Autodesk Inventor part; units mm, degrees
ref_plane "YZ Plane" through (0, 0, 0) normal (1, 0, 0) x (0, 1, 0)
ref_plane "XZ Plane" through (0, 0, 0) normal (0, 1, 0) x (-1, 0, 0)
ref_plane "XY Plane" through (0, 0, 0) normal (0, 0, 1) x (1, 0, 0)
ref_plane "Work Plane2" through (35.545, -31.609, 1.6) normal (0, 0, 1) x (1, 0, 0)
ref_plane "Work Plane1" through (35.545, -31.609, 1.6) normal (0, 0, 1) x (1, 0, 0)
sketch "Sketch1" plane through (35.545, -31.609, 1.6) normal (0, 0, 1) x (1, 0, 0)
  line L0 (0, 0) -> (336, 0)
  line L1 (-2, -129) -> (-2, -2)
  line L2 (-1.6825, -0.9187) -> (-1.5115, -0.6903)
  arc A0 (0, 0) -> (-2, -2) centre (0, -2) ccw
  line L3 (338, -2) -> (338, -129)
  line L4 (337.5115, -0.6903) -> (337.6825, -0.9187)
  arc A1 (338, -2) -> (336, 0) centre (336, -2) ccw
  line L5 (336, -131) -> (0, -131)
  line L6 (337.6825, -130.0813) -> (337.5115, -130.3097)
  arc A2 (336, -131) -> (338, -129) centre (336, -129) ccw
  arc A3 (-2, -129) -> (0, -131) centre (0, -129) ccw
  circle A4 centre (1.98, -128.63) radius 1.1
  circle A5 centre (1.98, -128.63) radius 1.1
  circle A6 centre (68.313, -128.63) radius 1.1
  circle A7 centre (134.646, -128.63) radius 1.1
  circle A8 centre (134.646, -128.63) radius 1.1
  circle A9 centre (68.313, -128.63) radius 1.1
  circle A10 centre (200.979, -128.63) radius 1.1
  circle A11 centre (267.312, -128.63) radius 1.1
  circle A12 centre (333.645, -128.63) radius 1.1
  circle A13 centre (333.645, -128.63) radius 1.1
  circle A14 centre (267.312, -128.63) radius 1.1
  circle A15 centre (200.979, -128.63) radius 1.1
  circle A16 centre (333.638, -2.355) radius 1.1
  circle A17 centre (1.973, -2.355) radius 1.1
  circle A18 centre (68.306, -2.355) radius 1.1
  circle A19 centre (134.639, -2.355) radius 1.1
  circle A20 centre (200.972, -2.355) radius 1.1
  circle A21 centre (267.305, -2.355) radius 1.1
  circle A22 centre (333.645, -2.355) radius 1.093
  circle A23 centre (267.305, -2.355) radius 1.1
  circle A24 centre (200.972, -2.355) radius 1.1
  circle A25 centre (134.639, -2.355) radius 1.1
  circle A26 centre (68.306, -2.355) radius 1.1
  circle A27 centre (1.973, -2.355) radius 1.1
  line L7 (3, -4.2357) -> (125.2758, -4.2357) construction
  line L8 (4, -5) -> (332, -5)
  line L9 (333, -6) -> (333, -125)
  line L10 (332, -126) -> (4, -126)
  line L11 (3, -125) -> (3, -6)
  arc A28 (4, -5) -> (3, -6) centre (4, -6) ccw
  arc A29 (333, -6) -> (332, -5) centre (332, -6) ccw
  arc A30 (332, -126) -> (333, -125) centre (332, -125) ccw
  arc A31 (3, -125) -> (4, -126) centre (4, -125) ccw
  line L12 (162.5077, 0) -> (162.5077, -5)
  line L13 (173.4174, -5) -> (173.4174, 0)
  circle A32 centre (320.737, -95.692) radius 0.175
  line L14 (333, -88.192) -> (338, -88.192)
  line L15 (333, -102.192) -> (338, -102.192)
  line L16 (257.6125, -126) -> (315.0362, -126)
  line L17 (315.0362, -126) -> (315.0362, -126.7604)
  line L18 (315.0362, -126.7604) -> (257.6125, -126.7604)
  line L19 (257.6125, -126.7604) -> (257.6125, -126)
  point P0 (-35.545, 31.609)
  point P1 (-1.5115, -130.3097)
  point P2 (335.5, -88.192)
  point P3 (0, -131)
  point P4 (337.6825, -130.0813)
  point P5 (-1.6825, -0.9187)
  point P6 (337.6825, -0.9187)
  dimension "d2" = 5
  dimension "d3" = 5
  dimension "d4" = 5
  dimension "d5" = 5
  dimension "d6" = 1
  dimension "d7" = 1
  dimension "d8" = 1
  dimension "d9" = 1
extrude "Extrusion3" add sketch "Sketch1" along normal blind 4.5 contours L0 A1 L4 L3 L14 L9 A29 L8 L13
properties part number "open_liner_S"
Here's how the part is built. I have some questions about the finished solid (model axes, mm). A direction names the side the tool comes from. Round coordinates to 2 decimals unless told otherwise and drop trailing zeros. Order: outer loops, then holes, each group sorted by start corner. A loop starts at its lowest first (then second) coordinate and runs counter-clockwise, first axis right, second up. Notation, with made-up numbers: M -4.5,17.25 L 3.5,17.25 A17 ccw 3.5,36.25 Z; hole C 77,-23.5 d6. An arc over 180 degrees is marked long. One line per question, with ' | ' between items.
1) I want a section at A-A, the plane z = 3.8. State how many separate pieces and enclosed holes the cut face has, then the cut area to 3 significant figures.
Working result:
separate pieces: 1 | enclosed holes: 3 | area: 1,230 mm²
2) I need wall thicknesses on line 1 along Y through (x, z) = (279, 4.9); line 2 along X through (y, z) = (-45, 3.5) (3 decimals). Which ranges of each line are inside material? Lowest first, please.
Working result:
line 1: -36.61 to -31.61 | line 2: 368.545 to 373.545
3) I want a section at B-B, the plane y = -93.5. Write out the boundary of the cut face in (x, z) (3 decimals).
Working result:
outline: M 368.545,1.6 L 373.545,1.6 L 373.545,6.1 L 368.545,6.1 Z
4) I want a section at C-C, the plane x = 265.5. Write out the boundary of the cut face in (y, z), then the cut area to 3 significant figures.
Working result:
outline: M -36.61,1.6 L -31.61,1.6 L -31.61,6.1 L -36.61,6.1 Z | area: 22.5 mm²
5) For faces 1 (the face through (368.545, -78, 4)), 2 (the face through (208.962, -34, 4)), which set-ups out of +Z, -Z, +X, -X, +Y, -Y let a thin tool reach every point of the face, with its end or its side?
Working result:
face 1: +Z, -Z, -X, -Y | face 2: +Z, -Z, -X, +Y, -Y
6) For pin 1 Ø1.3 at (x, z) = (281, 2.5) entering from -Y; pin 2 Ø2 at (y, z) = (-96.5, 4) entering from -X (3 decimals), each with a flat end and sliding along its axis, tell me the tip position at first contact or that it passes through.
Working result:
pin 1: y = -36.61 | pin 2: x = 368.545
